from build123d import *

# Parameters (mm, degrees)
F0_R     = 25
F0_R_2   = 7.5
F0_R_3   = 4
F1_DEPTH = 10
F2_R     = 25
F3_DEPTH = 2
F4_DEPTH = 25


with BuildPart() as f1:
    # F0 (on Front) → F1 (new body)
    with BuildSketch(Plane.XZ):
        Circle(F0_R)
        with Locations((0, -15)):
            Circle(F0_R_2, mode=Mode.SUBTRACT)
        with Locations((-12.990381, 7.5)):
            Circle(F0_R_2, mode=Mode.SUBTRACT)
        Circle(F0_R_3, mode=Mode.SUBTRACT)
        with Locations((12.990381, 7.5)):
            Circle(F0_R_2, mode=Mode.SUBTRACT)
    extrude(amount=-F1_DEPTH)

    # F2 (on face) → F3 (join)
    with BuildSketch(Plane(origin=(0, 10, 0), x_dir=(-1, 0, 0), z_dir=(0, 1, 0))):
        Circle(F2_R)
    extrude(amount=F3_DEPTH)

    # F0 (on Front) → F4 (cut)
    with BuildSketch(Plane.XZ):
        Circle(F0_R_3)
    extrude(amount=-F4_DEPTH, mode=Mode.SUBTRACT)


solid = f1.part
Input: part model. Units: mm. Frame: model coordinates. A direction names the side the tool comes from. Give positions to 0.01 mm unless a question says otherwise; leave off trailing zeros. Write each loop counter-clockwise with the first axis right and the second up, starting at its lowest first coordinate (ties: lowest second). Pieces come first, ordered by that corner, then holes.
Q1. Section A-A, the plane x = 0. Output: boundary loops of the cut face in (y, z), plus the area to 3 significant figures.
Q2. First-contact query: P1, Ø7.5, axis at x = -16.5, z = 7.5, coming from the -Y side; P2, Ø6, axis at y = 10.5, z = -17, coming from the +X side; P3, Ø3, axis at y = 8, z = 11, coming from the +X side; P4, Ø6.5, axis at x = 0, z = 0, coming from the -Y side. Flat tips, straight axial feed; report the tip coordinate or a pass-through.
Q3. Section D-D, the plane x = 17.5. Output: boundary loops of the cut face in (y, z).
Q4. Pull-direction query (X, two-part tool) for faces 3 (the face through (5, 0, 0)), 4 (the face through (0, 10, -15)); classes: pulls with the +X half, pulls with the -X half, needs draft (parallel to the pull), parting line crosses it, or undercut.
Q5. Section B-B, the plane z = -15. Output: boundary loops of the cut face in (x, y), plus the area to 3 significant figures.
Q6. Set-up query: faces 1 (the face through (0, 12, -5)), 2 (the face through (-9.53, 4.93, 0.846)). Return all of +Z, -Z, +X, -X, +Y, -Y with unobstructed straight access to the full face (end or side cutting, diameter ignored); none if empty.
Q7. Material intervals for probe 1 along Z at (x, y) = (0, 2.5); probe 2 along X at (y, z) = (7.25, 5.5); probe 3 along Z at (x, y) = (-3, 5.25), sorted ascending.
Q8. Section C-C, the plane y = 8.75. Output: boundary loops of the cut face in (x, z).
Filled in:
1. outline: (0, -25) - (12, -25) - (12, -4) - (0, -4) - (0, -7.5) - (10, -7.5) - (10, -22.5) - (0, -22.5) - close; (0, 4) - (12, 4) - (12, 25) - (0, 25) - close
1. area: 354 mm2
2. P1: stops at y = 10
2. P2: stops at x = 20.71
2. P3: stops at x = 23.12
2. P4: passes through
3. outline: (0, -17.85) - (12, -17.85) - (12, 17.85) - (0, 17.85) - (0, 13.49) - (10, 13.49) - (10, 1.51) - (0, 1.51) - close
4. face 3: needs draft
4. face 4: undercut
5. outline: (-20, 0) - (-7.5, 0) - (-7.5, 10) - (7.5, 10) - (7.5, 0) - (20, 0) - (20, 12) - (-20, 12) - close
5. area: 330 mm2
6. face 1: +Z, -Z, +X, -X, +Y
6. face 2: -Y
7. probe 1: z = -25 to -22.5, -7.5 to -4, 4 to 25
7. probe 2: x = -24.39 to -20.22, -5.76 to 5.76, 20.22 to 24.39
7. probe 3: z = -24.82 to -21.87, -8.13 to -2.65, 2.65 to 24.82
8. outline: circle Ø50 at (0, 0); hole circle Ø15 at (-12.99, 7.5); hole circle Ø15 at (0, -15); hole circle Ø8 at (0, 0); hole circle Ø15 at (12.99, 7.5)
